Here's how the part is built. I have some questions about the finished solid (model axes, mm). Give positions to 0.01 mm unless a question says otherwise; leave off trailing zeros. Write each loop counter-clockwise with the first axis right and the second up, starting at its lowest first coordinate (ties: lowest second). Pieces come first, ordered by that corner, then holes. Notation, with made-up numbers: (75.25, 49) -> (129.25, 49) arc R18 cw to (129.25, 82) -> close; hole circle Ø9 at (8, 2.25). An arc over 180 degrees is marked (long way). Use one line per item in the form item = value.
```python
from build123d import *

# Parameters (mm, degrees)
SKETCH1_W                       = 127
SKETCH1_H                       = 65
EXTRUDE1_DEPTH                  = 6.35
M6X1_0_TAPPED_HOLE1_D           = 5
CBORE_FOR_M6_SBHCS1_D           = 7
CBORE_FOR_M6_SBHCS1_CBORE_D     = 11.5
CBORE_FOR_M6_SBHCS1_CBORE_DEPTH = 3.3


with BuildPart() as part:
    # Sketch1 → Extrude1 (new body)
    with BuildSketch(Plane(origin=(0, 0, 0), x_dir=(1, 0, 0), z_dir=(0, 1, 0))):
        Rectangle(SKETCH1_W, SKETCH1_H)
    extrude(amount=EXTRUDE1_DEPTH)

    # M6x1.0 Tapped Hole1 (through all)
    with Locations(Plane(origin=(0, 6.35, 0), x_dir=(-1, 0, 0), z_dir=(0, 1, 0))):
        with Locations((-42.5, -12.6), (-42.5, 12.6)):
            Hole(M6X1_0_TAPPED_HOLE1_D / 2)

    # CBORE for M6 SBHCS1 (through all)
    with Locations(Plane.XZ):
        with Locations((-44, 12.5), (-19, 12.5), (-19, -12.5), (-44, -12.5)):
            CounterBoreHole(CBORE_FOR_M6_SBHCS1_D / 2, CBORE_FOR_M6_SBHCS1_CBORE_D / 2, CBORE_FOR_M6_SBHCS1_CBORE_DEPTH)


solid = part.part
```
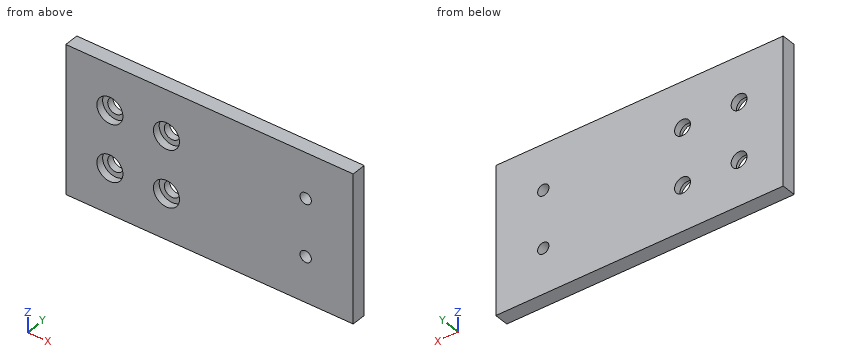
Q1. Will this pin go through, and if not, where does the flat tip stop? pin 1 Ø6 at (x, z) = (-45, 12) entering from -Y.
Result set:
pin_1 = 3.3
Q2. I want a section at A-A, the plane x = -19. Write out the boundary of the cut face in (y, z).
Result set:
outline = (0, -32.5) -> (6.35, -32.5) -> (6.35, -16) -> (3.3, -16) -> (3.3, -18.25) -> (0, -18.25) -> close; (0, -6.75) -> (3.3, -6.75) -> (3.3, -9) -> (6.35, -9) -> (6.35, 9) -> (3.3, 9) -> (3.3, 6.75) -> (0, 6.75) -> close; (0, 18.25) -> (3.3, 18.25) -> (3.3, 16) -> (6.35, 16) -> (6.35, 32.5) -> (0, 32.5) -> close
Q3. If I drill on line 1 along Z through (x, y) = (-19, 5.45); line 2 along Z through (x, y) = (-44, 2.1); line 3 along Y through (x, z) = (-47.5, -14), over which ranges is the centre line in solid material (lowest first)? Write a range as from..to.
Result set:
line_1 = -32.5..-16, -9..9, 16..32.5
line_2 = -32.5..-18.25, -6.75..6.75, 18.25..32.5
line_3 = 3.3..6.35
